```python
from build123d import *

# Parameters (mm, degrees)
BOSS_EXTRUDE1_DEPTH = 285.75
SKETCH2_R           = 3.175
CUT_EXTRUDE1_DEPTH  = 292.961923887
SKETCH3_R           = 1.4224
CUT_EXTRUDE2_DEPTH  = 6.35
SKETCH4_R           = 3.175
CUT_EXTRUDE3_DEPTH  = 292.961923887


with BuildPart() as part:
    # Sketch1 → Boss-Extrude1 (new body)
    with BuildSketch(Plane(origin=(0, 0, 0), x_dir=(0, 0, -1), z_dir=(1, 0, 0))):
        Polygon((-19.05, -31.75), (-19.05, -4.7625), (19.05, -4.7625), (19.05, -31.75), (25.4, -31.75), (25.4, 0), (-25.4, 0), (-25.4, -31.75), align=None)
    extrude(amount=BOSS_EXTRUDE1_DEPTH)

    # Sketch2 → Cut-Extrude1 (cut, through all)
    with BuildSketch(Plane.XY.offset(25.4)):
        with Locations((9.525, -18.415)):
            Circle(SKETCH2_R)
        with Locations((79.068028046, -19.05)):
            Circle(SKETCH2_R)
        with Locations((117.168028046, -19.05)):
            Circle(SKETCH2_R)
        with Locations((155.268028046, -19.05)):
            Circle(SKETCH2_R)
        with BuildLine():
            Line((206.375, -11.1125), (257.175, -11.1125))
            ThreePointArc((257.175, -11.1125), (261.9375, -15.875), (257.175, -20.6375))
            Line((257.175, -20.6375), (206.375, -20.6375))
            ThreePointArc((206.375, -20.6375), (201.6125, -15.875), (206.375, -11.1125))
        make_face()
    extrude(amount=-CUT_EXTRUDE1_DEPTH, mode=Mode.SUBTRACT)

    # Sketch3 → Cut-Extrude2 (cut)
    with BuildSketch(Plane(origin=(0, 0, 0), x_dir=(1, 0, 0), z_dir=(0, 1, 0))):
        with Locations(Location((147.7645, 14.2875, 0), (0, 0, 270))):
            Circle(SKETCH3_R)
        with Locations(Location((147.7645, -14.2875, 0), (0, 0, 270))):
            Circle(SKETCH3_R)
        with BuildLine():
            Line((196.85, 7.14375), (266.7, 7.14375))
            ThreePointArc((266.7, 7.14375), (273.84375, 0), (266.7, -7.14375))
            Line((266.7, -7.14375), (196.85, -7.14375))
            ThreePointArc((196.85, -7.14375), (189.70625, 0), (196.85, 7.14375))
        make_face()
    extrude(amount=-CUT_EXTRUDE2_DEPTH, mode=Mode.SUBTRACT)

    # Sketch4 → Cut-Extrude3 (cut, through all)
    with BuildSketch(Plane.XY.offset(25.4)):
        with Locations((273.05, -15.875)):
            Circle(SKETCH4_R)
    extrude(amount=-CUT_EXTRUDE3_DEPTH, mode=Mode.SUBTRACT)


solid = part.part
```
Check sheet for the modelled part. Datum: model origin and axes. Units: mm. A direction names the side the tool comes from. Round coordinates to 2 decimals unless told otherwise and drop trailing zeros. Order: outer loops, then holes, each group sorted by start corner. A loop starts at its lowest first (then second) coordinate and runs counter-clockwise, first axis right, second up.
1) Section check C-C (x = 63.5). Record the boundary of the cut face in (y, z).
2) Tool access check on faces 5 (the flat face through (232, -20.638, 22)), 6 (the flat face through (231, -2, -7.144)), 7 (the flat face through (0, -4, 0)). Record the directions out of +Z, -Z, +X, -X, +Y, -Y that give a thin tool (end or side, any length) a straight path to the whole face; none if there is none.
3) Go/stop test with flat-tipped pins: pin 1 Ø8.5 at (x, y) = (79.07, -19.05) entering from -Z; pin 2 Ø5 at (x, y) = (9.525, -18.415) entering from -Z; pin 3 Ø12 at (x, z) = (254, -11) entering from -Y. Record where each tip stops, or that it passes through.
4) Section check D-D (z = 22.5). Give the number of separate pieces and of enclosed holes in the cut face, and give its area (3 significant figures).
5) Scan lines: line 1 (Z direction, x = 196, y = -6); line 2 (Y direction, x = 273, z = -22). Record each from-to range of solid material in increasing order.
6) Section check A-A (x = 245). Record the boundary of the cut face in (y, z), and give its area (3 significant figures).
7) Mould release check, pull along Z, two halves, no side actions. Record for faces 1 (the cylindrical face through (152.096, -18.91, 22.269)), 2 (the flat face through (141, -16, -25.4)), 3 (the flat face through (141, -16, 25.4)), 4 (the flat face through (232, -2, 7.144)): +Z half, -Z half, draft (parallel to the pull), parting line (faces both ways), or undercut.
8) Section check B-B (z = -4.5). Record the boundary of the cut face in (x, y), and give its area (3 significant figures).
Result:
1. outline: (-31.75, -25.4) - (0, -25.4) - (0, 25.4) - (-31.75, 25.4) - (-31.75, 19.05) - (-4.76, 19.05) - (-4.76, -19.05) - (-31.75, -19.05) - close
2. face 5: +Z, -Z
2. face 6: +Y, -Y
2. face 7: +Z, -Z, -X, +Y, -Y
3. pin 1: stops at z = -25.4
3. pin 2: passes through
3. pin 3: stops at y = -4.76
4. separate pieces: 1
4. enclosed holes: 6
4. area: 8,360 mm2
5. line 1: z = -25.4 to -19.05, 19.05 to 25.4
5. line 2: y = -31.75 to -19.05, -12.7 to 0
6. outline: (-31.75, -25.4) - (-20.64, -25.4) - (-20.64, -19.05) - (-31.75, -19.05) - close; (-31.75, 19.05) - (-20.64, 19.05) - (-20.64, 25.4) - (-31.75, 25.4) - close; (-11.11, -25.4) - (0, -25.4) - (0, -7.14) - (-4.76, -7.14) - (-4.76, -19.05) - (-11.11, -19.05) - close; (-11.11, 19.05) - (-4.76, 19.05) - (-4.76, 7.14) - (0, 7.14) - (0, 25.4) - (-11.11, 25.4) - close
6. area: 396 mm2
7. face 1: draft
7. face 2: -Z half
7. face 3: +Z half
7. face 4: undercut
8. outline: (0, -4.76) - (191.3, -4.76) - (191.3, 0) - (0, 0) - close; (272.25, -4.76) - (285.75, -4.76) - (285.75, 0) - (272.25, 0) - close
8. area: 975 mm2
